Read the model definition and answer for the solid it produces. Units are mm, in the model's axes. A direction names the side the tool comes from. Coordinates: 2 decimals unless noted, no trailing zeros. Write each loop counter-clockwise with the first axis right and the second up, starting at its lowest first coordinate (ties: lowest second). Pieces come first, ordered by that corner, then holes. Notation, with made-up numbers: (29, -29) -> (56, -29) arc R12 ccw to (56, -17) -> close; hole circle Ø10 at (-26.75, -21). An arc over 180 degrees is marked (long way). Answer as a JSON object with one key per item and string values. Group by question number.
(1) Find section C-C (y = 37). Count the separate pieces of the cut face and the enclosed holes in it, then the cut area to 3 significant figures.
(2) Find section B-B (z = -50). Give the vertices of the cut face in (x, y).
(3) Flat-ended cylindrical pins translate along their axes: P1, Ø14.5, axis at x = 15, z = 27.5, coming from the -Y side; P2, Ø4, axis at x = -27.5, z = -103.5, coming from the +Y side; P3, Ø8.5, axis at y = 25, z = 50, coming from the +X side. Find the tip coordinate at first contact, or state that the pin passes through.
(4) Find section A-A (y = 25). Give the vertices of the cut face in (x, z), then the cut area to 3 significant figures.
(5) For a pull along Z with two mould halves and no side action, classify faces 6 (the face through (-10, 25, 112.5)), 7 (the face through (0, 50, 2)), 8 (the face through (11.45, 32.75, -23.63)) as +Z half, -Z half, draft (parallel to the pull), parting line (faces both ways), or undercut.
(6) Straight lines are drawn through the part: L1, parallel to Z at x = -27.5, y = 38.75; L2, parallel to X at y = 37, z = -27.5; L3, parallel to Z at x = 13, y = 4. For each, find the intervals that lie inside material, in ascending order.
(7) Find section D-D (x = -5.5). Give the vertices of the cut face in (y, z), then the cut area to 3 significant figures.
(8) Which of the six approach directions +Z, -Z, +X, -X, +Y, -Y give full straight-line access (tool end or side, diameter ignored) to faces 1 (the face through (0, 29, -54)), 2 (the face through (-17.74, 28.19, -45.83)), 3 (the face through (0, 0, 2)), 4 (the face through (-30.8, 42.4, 76.1)), 5 (the face through (18.9, 15, 23.6))?
Autodesk Inventor part; units mm, degrees
ref_plane "YZ Plane" through (0, 0, 0) normal (1, 0, 0) x (0, 1, 0)
ref_plane "XZ Plane" through (0, 0, 0) normal (0, 1, 0) x (-1, 0, 0)
ref_plane "XY Plane" through (0, 0, 0) normal (0, 0, 1) x (1, 0, 0)
sketch "Sketch1" plane through (0, 0, 0) normal (0, 1, 0) x (-1, 0, 0)
  line L0 (35, 112.5) -> (-35, 112.5)
  line L1 (-35, 112.5) -> (-35, -112.5)
  line L2 (-35, -112.5) -> (35, -112.5)
  line L3 (35, -112.5) -> (35, 112.5)
  point P0 (0, 0)
  point P1 (35, 0)
  point P2 (0, -112.5)
  dimension "d0" = 225
  dimension "d1" = 70
extrude "Extrusion1" add sketch "Sketch1" along normal blind 50
sketch "Sketch2" plane through (35, 0, 112.5) normal (1, 0, 0) x (0, 0, -1)
  circle A0 centre (62.5, 25) radius 5
  circle A1 centre (162.5, 25) radius 5
  line L0 (225, 0) -> (225, 50)
  point P0 (0, 50)
  point P1 (112.5, 0)
  point P2 (225, 25)
  dimension "d5" = 50
  dimension "d6" = 50
  dimension "d8" = 225
  dimension "d33" = 10
hole "Hole1" at (35, 25, 50) at (35, 25, -50) direction (-1, 0, 0) diameter 10.5 end through all counterbore diameter 18 counterbore depth 35
sketch "Sketch3" plane through (0, 0, 0) normal (0, -1, 0) x (1, 0, 0)
  line L0 (35, 112.5) -> (35, -112.5)
  circle A0 centre (15, 27.5) radius 5
  circle A1 centre (15, -27.5) radius 5
  point P0 (0, 0)
  dimension "d17" = 55
  dimension "d18" = 20
  dimension "d21" = 27.5
  dimension "d32" = 10
hole "Hole2" at (15, 0, 27.5) at (15, 0, -27.5) direction (0, 1, 0) diameter 10.5 end through all counterbore diameter 18 counterbore depth 15
chamfer "Chamfer1" distance 20 angle 45 2 edges at (35, 25, 112.5) (35, 25, -112.5)
sketch "Sketch4" plane through (0, 50, 0) normal (0, 1, 0) x (1, 0, 0)
  line L0 (-35, 112.5) -> (-35, -112.5)
  circle A0 centre (-27.5, -103.5) radius 4
  circle A1 centre (-27.5, -76.5) radius 4
  circle A2 centre (-14, -90) radius 4
  line L1 (0, 0) -> (7.2062, 0) construction
  circle A3 centre (-27.5, 103.5) radius 4
  circle A4 centre (-27.5, 76.5) radius 4
  circle A5 centre (-14, 90) radius 4
  dimension "d36" = 13.5
  dimension "d37" = 27
  dimension "d38" = 8
  dimension "d39" = 7.5
  dimension "d40" = 8
  dimension "d41" = 90
  dimension "d42" = 13.5
hole "Hole3" at (-27.5, 50, 103.5) at (-14, 50, 90) at (-27.5, 50, 76.5) at (-27.5, 50, -76.5) at (-14, 50, -90) at (-27.5, 50, -103.5) direction (0, -1, 0) diameter 6.647 depth 15 tip angle 118
chamfer "Chamfer2" distance 1 angle 45 10 edges at (-10, 50, 112.5) (25, 50, 102.5) (35, 50, 0) (25, 50, -102.5) (-10, 50, -112.5) (-10, 0, 112.5) (25, 0, 102.5) (35, 0, 0) (25, 0, -102.5) (-10, 0, -112.5)
properties part number "BC-10008" material "Aço Carbono AISI 1006"
Results below:
{
 "1": {"separate pieces": "1", "enclosed holes": "8", "area": "15,000 mm2"},
 "2": {"outline": "(-35, 0) -> (34, 0) -> (35, 1) -> (35, 16) -> (0, 16) -> (0, 19.75) -> (-35, 19.75) -> close; (-35, 30.25) -> (0, 30.25) -> (0, 34) -> (35, 34) -> (35, 49) -> (34, 50) -> (-35, 50) -> close"},
 "3": {"P1": "stops at y = 15", "P2": "stops at y = 34.2", "P3": "passes through"},
 "4": {"outline": "(-35, -112.5) -> (15, -112.5) -> (35, -92.5) -> (35, -59) -> (0, -59) -> (0, -55.25) -> (-35, -55.25) -> close; (-35, -44.75) -> (0, -44.75) -> (0, -41) -> (35, -41) -> (35, 41) -> (0, 41) -> (0, 44.75) -> (-35, 44.75) -> close; (-35, 55.25) -> (0, 55.25) -> (0, 59) -> (35, 59) -> (35, 92.5) -> (15, 112.5) -> (-35, 112.5) -> close; hole circle Ø10.5 at (15, -27.5); hole circle Ø10.5 at (15, 27.5)", "area": "13,200 mm2"},
 "5": {"face 6": "+Z half", "face 7": "draft", "face 8": "undercut"},
 "6": {"L1": "z = -112.5 to -106.82, -100.18 to -79.82, -73.18 to 73.18, 79.82 to 100.18, 106.82 to 112.5", "L2": "x = -35 to 9.75, 20.25 to 35", "L3": "z = -112.5 to -36.27, -18.73 to 18.73, 36.27 to 112.5"},
 "7": {"outline": "(0, -111.5) -> (1, -112.5) -> (49, -112.5) -> (50, -111.5) -> (50, 111.5) -> (49, 112.5) -> (1, 112.5) -> (0, 111.5) -> close; hole circle Ø10.5 at (25, -50); hole circle Ø10.5 at (25, 50)", "area": "11,100 mm2"},
 "8": {"face 1": "+X", "face 2": "+X, -X", "face 3": "+Z, -Z, +X, -X, -Y", "face 4": "+Y", "face 5": "-Y"}
}
